Design review of the part built by this model. Coordinates are the model's own, in mm. A direction names the side the tool comes from. Round coordinates to 2 decimals unless told otherwise and drop trailing zeros. Loops run counter-clockwise (first coordinate to the right, second up) from the corner with the lowest first, then second, coordinate; pieces in that order, holes last. Notation, with made-up numbers: (20, 57.25) - (34, 57.25) arc R34 cw to (34, 95.25) - close; hole circle Ø4 at (73.5, 46). An arc over 180 degrees is marked (long way). Return JSON: item names as keys, results as strings. Group by question number.
(1) We need section B-B, the plane z = -26.5. Write out the cut boundary in (x, y), and give its area (3 significant figures).
(2) For faces 4 (the cylindrical face through (2.285, 3.584, 2.366)), 5 (the flat face through (1.4, -1.43, 3.77)), list the 3-axis set-ups (+Z, -Z, +X, -X, +Y, -Y) from which the entire face can be reached by the end or side of a thin tool; tool diameter is ignored.
(3) We need section A-A, the plane x = 0. Write out the cut boundary in (y, z).
(4) The part is to be moulded in two halves that separate along X. For faces 1 (the flat face through (2, -2, 0)), 2 (the cylindrical face through (-2.5, -0.1, -17.3)), 3 (the flat face through (-1.4, 1.43, 3.77)), say which applies: pulls with the +X half, pulls with the -X half, needs draft (parallel to the pull), parting line crosses it, or undercut.
(5) Clearance check with flat-ended pins moving along their axes: pin 1 (3 mm diameter, centred on y = 0, z = -27.5, fed in from +X); pin 2 (1.5 mm diameter, centred on x = -0.5, z = -5, fed in from -Y); pin 3 (3 mm diameter, centred on y = -0.5, z = -6, fed in from -X); pin 4 (3.5 mm diameter, centred on x = 0.5, y = 1, fed in from +Z). State where each tip first meets the part, or that it passes through.
(6) Wall thickness on L1, parallel to Z at x = 0.25, y = 1; L2, parallel to Z at x = -1.25, y = -3.5; L3, parallel to X at y = 2, z = -11.5: over which ranges is each line inside the solid? List them lowest first. Write a range as [from, to].
from build123d import *

# Parameters (mm, degrees)
SKETCH_1_R          = 4.25
EXTRUDE_1_DEPTH     = 5
CUT_EXTRUDE_1_DEPTH = 2.5
SKETCH_3_R          = 2.5
EXTRUDE_2_DEPTH     = 35
FILLET_1_R          = 0.2


with BuildPart() as part:
    # 草图1 → 凸台-拉伸1 (new body)
    with BuildSketch(Plane.XY):
        Circle(SKETCH_1_R)
    extrude(amount=EXTRUDE_1_DEPTH)

    # 草图2 → 切除-拉伸1 (cut)
    with BuildSketch(Plane.XY.offset(5)):
        Polygon((-1.632993162, -1.632993162), (0.597716981, -2.230710143), (2.230710143, -0.597716981), (1.632993162, 1.632993162), (-0.597716981, 2.230710143), (-2.230710143, 0.597716981), align=None)
    extrude(amount=-CUT_EXTRUDE_1_DEPTH, mode=Mode.SUBTRACT)

    # 草图3 → 凸台-拉伸2 (add)
    with BuildSketch(Plane(origin=(0, 0, 0), x_dir=(-1, 0, 0), z_dir=(0, 0, -1))):
        with Locations(Location((0, 0, 0), (0, 0, 180))):
            Circle(SKETCH_3_R)
    extrude(amount=EXTRUDE_2_DEPTH)

    # 圆角1
    fillet_1_edges = [part.edges().sort_by_distance(p)[0] for p in [
        (-4.25, 0, 5),
    ]]
    fillet(fillet_1_edges, radius=FILLET_1_R)


solid = part.part
Solutions:
{
 "1": {"outline": "circle Ø5 at (0, 0)", "area": "19.6 mm^2"},
 "2": {"face 4": "+Z, -Z", "face 5": "+Z"},
 "3": {"outline": "(-4.25, 0) - (-2.5, 0) - (-2.5, -35) - (2.5, -35) - (2.5, 0) - (4.25, 0) - (4.25, 4.8) arc R0.2 ccw to (4.05, 5) - (2.07, 5) - (2.07, 2.5) - (-2.07, 2.5) - (-2.07, 5) - (-4.05, 5) arc R0.2 ccw to (-4.25, 4.8) - close"},
 "4": {"face 1": "needs draft", "face 2": "parting line crosses it", "face 3": "undercut"},
 "5": {"pin 1": "x = 2.5", "pin 2": "y = -2.5", "pin 3": "x = -2.5", "pin 4": "z = 5"},
 "6": {"L1": "[-35, 2.5]", "L2": "[0, 5]", "L3": "[-1.5, 1.5]"}
}
